Answer from the drawing. Dimensions are ordinates in mm from the lowest x, y and z of the part. A direction names the side the tool comes from. Give positions to 0.01 mm unless a question says otherwise; leave off trailing zeros. Order: outer loops, then holes, each group sorted by start corner. A loop starts at its lowest first (then second) coordinate and runs counter-clockwise, first axis right, second up. Notation, with made-up numbers: (-26.75, -16) - (-21.75, -16) arc R20 cw to (-21.75, 13) - close; hole circle Ø8 at (35, 36.5). An arc over 180 degrees is marked (long way). Use a Markdown table: item, result. Add a question column.
1) Find section C-C, the plane z = 11.5. Determine the outline of the cut face in (x, y), plus the area to 3 significant figures.
2) Straight lines are drawn through the part: line 1 (X direction, y = 12, z = 4); line 2 (X direction, y = 6, z = 13.5); line 3 (Z direction, x = 9.5, y = 8). For each, find the intervals that lie inside material, in ascending order.
3) Find section D-D, the plane y = 5.5. Determine the outline of the cut face in (x, z), plus the area to 3 significant figures.
4) Find section B-B, the plane y = 9.75. Determine the outline of the cut face in (x, z), plus the area to 3 significant figures.
5) For the marked faces 1, 2, 3, 4 and 5, determine the directions among +Z, -Z, +X, -X, +Y, -Y from which every point of the face is accessible in a straight line to the end or side of a thin tool.
6) Find section A-A, the plane x = 33. Determine the outline of the cut face in (y, z), plus the area to 3 significant figures.
7) The mould has two halves that part along Z. Classify the marked faces 6, 7 and 8: released by +Z, released by -Z, zero draft, split by the parting line, or undercut.
8) Flat-ended cylindrical pins translate along their axes: pin 1 (0.8 mm diameter, centred on x = 25, z = 8.5, fed in from -Y); pin 2 (6.5 mm diameter, centred on x = 39.5, y = 7, fed in from +Z); pin 3 (5 mm diameter, centred on y = 9.5, z = 18.5, fed in from +X); pin 4 (5.5 mm diameter, centred on y = 8.5, z = 21.5, fed in from +X). Find the tip coordinate at first contact, or state that the pin passes through.
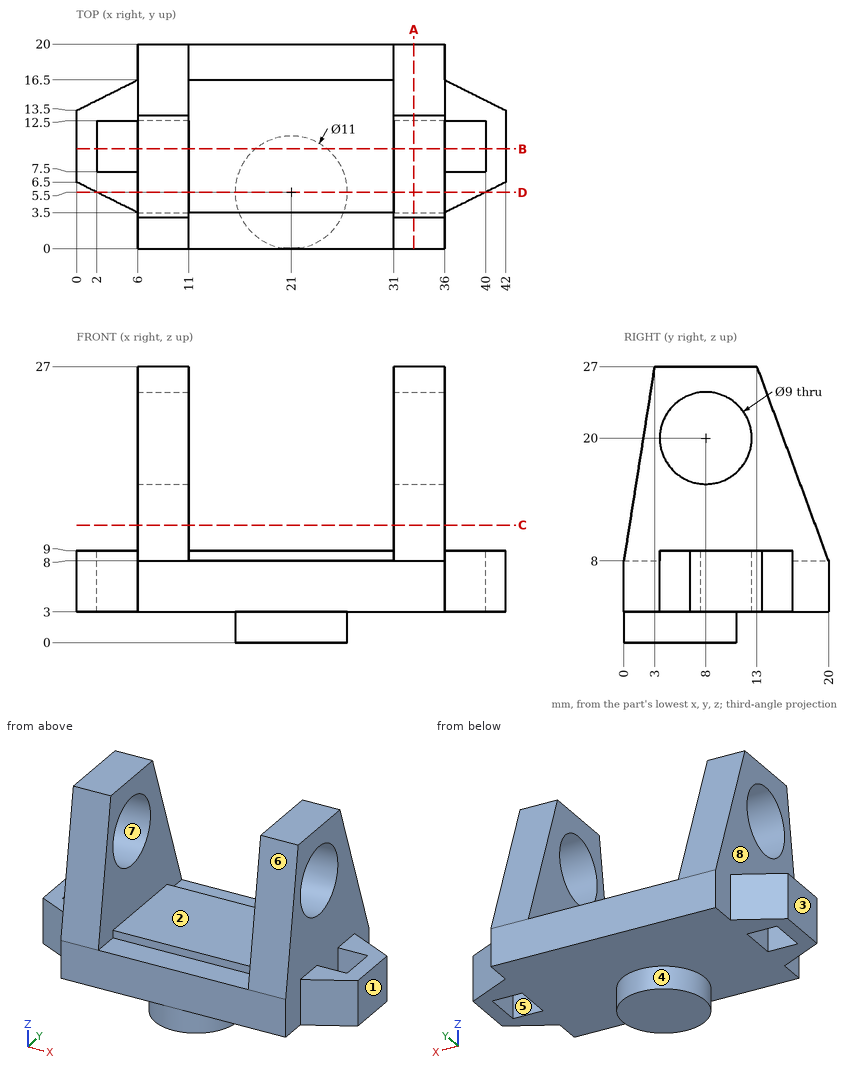
The answers:
| question | item | result |
|---|---|---|
| 1 | outline | (6, 0.55) - (11, 0.55) - (11, 18.71) - (6, 18.71) - close; (31, 0.55) - (36, 0.55) - (36, 18.71) - (31, 18.71) - close |
| 1 | area | 182 mm2 |
| 2 | line 1 | 0 to 2, 6 to 36, 40 to 42 |
| 2 | line 2 | 6 to 11, 31 to 36 |
| 2 | line 3 | 3 to 15.5, 24.5 to 27 |
| 3 | outline | (2, 3) - (15.5, 3) - (15.5, 0) - (26.5, 0) - (26.5, 3) - (40, 3) - (40, 9) - (36, 9) - (36, 16.26) - (31, 16.26) - (31, 9) - (11, 9) - (11, 16.26) - (6, 16.26) - (6, 9) - (2, 9) - close; (6, 23.74) - (11, 23.74) - (11, 27) - (6, 27) - close; (31, 23.74) - (36, 23.74) - (36, 27) - (31, 27) - close |
| 3 | area | 366 mm2 |
| 4 | outline | (0, 3) - (2, 3) - (2, 9) - (0, 9) - close; (6, 3) - (17.51, 3) - (17.51, 0) - (24.49, 0) - (24.49, 3) - (36, 3) - (36, 15.85) - (31, 15.85) - (31, 9) - (11, 9) - (11, 15.85) - (6, 15.85) - close; (6, 24.15) - (11, 24.15) - (11, 27) - (6, 27) - close; (31, 24.15) - (36, 24.15) - (36, 27) - (31, 27) - close; (40, 3) - (42, 3) - (42, 9) - (40, 9) - close |
| 4 | area | 322 mm2 |
| 5 | face 1 | +Z, -Z, +X, +Y, -Y |
| 5 | face 2 | +Z, +Y, -Y |
| 5 | face 3 | +Z, -Z, -X, +Y, -Y |
| 5 | face 4 | -Z |
| 5 | face 5 | +Z, -Z |
| 6 | outline | (0, 3) - (20, 3) - (20, 8) - (13, 27) - (3, 27) - (0, 8) - close; hole circle Ø9 at (8, 20) |
| 6 | area | 321 mm2 |
| 7 | face 6 | released by +Z |
| 7 | face 7 | undercut |
| 7 | face 8 | zero draft |
| 8 | pin 1 | y = 3.5 |
| 8 | pin 2 | z = 9 |
| 8 | pin 3 | x = 36 |
| 8 | pin 4 | through |
